```python
from build123d import *

# Parameters (mm, degrees)
F0_W          = 6
F0_H          = 3
F1_DEPTH      = 6
F2_DEPTH      = 2
F2_DEPTH_BACK = 3
F3_R          = 1.7
F4_DEPTH      = 4.8
F5_R          = 2
F6_R          = 1.7
F7_DEPTH      = 3


with BuildPart() as f1:
    # F0 (on Front) → F1 (new body, symmetric)
    with BuildSketch(Plane.XZ):
        with BuildLine():
            Line((10, 0), (22.5, 0))
            Line((22.5, 0), (18.9995524919, 20.0000000164))
            Line((18.9995524919, 20.0000000164), (18.9995524919, 25.5000000164))
            Line((18.9995524919, 25.5000000164), (8.0836130781, 25.5000000164))
            ThreePointArc((8.0836130781, 25.5000000164), (5.5476302699, 20.0983556377), (0, 17.8999996185))
            Line((0, 17.8999996185), (0, 15.5))
            Line((0, 15.5), (10, 15.5))
            Line((10, 15.5), (10, 0))
        make_face()
        with Locations((12.9995524922, 19.0000000164)):
            Rectangle(F0_W, F0_H, mode=Mode.SUBTRACT)
    extrude(amount=F1_DEPTH, both=True)

    # F0 (on Front) → F2 (join, two sides)
    with BuildSketch(Plane.XZ) as f2_sk:
        with BuildLine():
            ThreePointArc((0, 17.8999996185), (5.5476302699, 20.0983556377), (8.0836130781, 25.5000000164))
            Line((8.0836130781, 25.5000000164), (6.0785524919, 25.5000000164))
            ThreePointArc((6.0785524919, 25.5000000164), (4.1324570431, 21.5134004627), (0, 19.8999996185))
            Line((0, 19.8999996185), (0, 17.8999996185))
        make_face()
    extrude(amount=F2_DEPTH)
    extrude(f2_sk.sketch, amount=-F2_DEPTH_BACK)

    # F3 (on face) → F4 (cut)
    with BuildSketch(Plane.XY.offset(25.5000000164)):
        with Locations((12.9995524919, 0)):
            Circle(F3_R)
    extrude(amount=-F4_DEPTH, mode=Mode.SUBTRACT)

    # F5
    f5_edges = [f1.edges().sort_by_distance(p)[0] for p in [
        (20.749776, 6, 10),
        (18.999552, 6, 22.75),
        (20.749776, -6, 10),
        (18.999552, -6, 22.75),
    ]]
    fillet(f5_edges, radius=F5_R)

    # F6 (on face) → F7 (cut)
    with BuildSketch(Plane.XY.offset(17.5000000164)):
        with Locations((12.9995524922, 0)):
            Circle(F6_R)
    extrude(amount=-F7_DEPTH, mode=Mode.SUBTRACT)

    # F8: F1 across plane


with BuildPart() as f1_1:
    add(f1.part)
    add(f1.part.mirror(Plane.YZ))


solid = f1_1.part
```
Here's how the part is built. I have some questions about the finished solid (model axes, mm). A direction names the side the tool comes from. Coordinates: 2 decimals unless noted, no trailing zeros. Order: outer loops, then holes, each group sorted by start corner. A loop starts at its lowest first (then second) coordinate and runs counter-clockwise, first axis right, second up. Notation, with made-up numbers: M 17.5,78.25 L 39.5,78.25 A18 ccw 39.5,86.25 Z; hole C 39,-16 d11. An arc over 180 degrees is marked long. Answer as a JSON object with one key per item and string values. Group by question number.
(1) Suppose I cut it at C-C, the plane x = -5. Please give me the cut outline in (y, z), then the cut area to 3 significant figures.
(2) For pin 1 (1.7 mm diameter, centred on x = -13, y = -0.5, fed in from +Z); pin 2 (0.9 mm diameter, centred on y = -0.5, z = 19.5, fed in from -X); pin 3 (1 mm diameter, centred on x = -0.5, y = 0, fed in from +Z); pin 4 (3.5 mm diameter, centred on x = 12.5, y = 0.5, fed in from +Z), each with a flat end and sliding along its axis, tell me the tip position at first contact or that it passes through.
(3) Suppose I cut it at D-D, the plane y = 4.5. Please give me the cut outline in (x, z), then the cut area to 3 significant figures.
(4) Suppose I cut it at A-A, the plane y = -2.75. Please give me the cut outline in (x, z), then the cut area to 3 significant figures.
(5) Suppose I cut it at B-B, the plane z = 22.75. Please give me the cut outline in (x, y), then the cut area to 3 significant figures.
(6) Which directions (+Z, -Z, +X, -X, +Y, -Y) give clear straight access to the entire face, cutting with the end or side of a thin tool? Please do faces 1 (the face through (-13, 0, 14.5)), 2 (the face through (0, -2, 19)), 3 (the face through (10, 0, 8)), 4 (the face through (-16, 0, 19)), 5 (the face through (-19, 0, 23)).
(7) If we mould it in two halves opening along Y, with no side actions, what happens to faces 6 (the face through (20.12, 5.43, 10.12)), 7 (the face through (16, 0, 0)), 8 (the face through (13, 0, 20.7))? For each: released by +Y, released by -Y, zero draft, split by the parting line, or undercut.
(8) I need wall thicknesses on probe 1 along Z at (x, y) = (13, 5); probe 2 along X at (y, z) = (1.5, 15); probe 3 along X at (y, z) = (0.25, 22). Which ranges of each line are inside material? Lowest first, please.
Values found:
{
 "1": {"outline": "M -6,15.5 L 6,15.5 L 6,19.63 L 3,19.63 L 3,22.51 L -2,22.51 L -2,19.63 L -6,19.63 Z", "area": "63.9 mm^2"},
 "2": {"pin 1": "stops at z = 20.7", "pin 2": "stops at x = -19.17", "pin 3": "stops at z = 19.98", "pin 4": "stops at z = 25.5"},
 "3": {"outline": "M -22.44,0 L -10,0 L -10,15.5 L 10,15.5 L 10,0 L 22.44,0 L 18.94,19.99 L 18.94,25.5 L 8.08,25.5 A8.1 cw -8.08,25.5 L -18.94,25.5 L -18.94,19.99 Z; hole M -16,17.5 L -10,17.5 L -10,20.5 L -16,20.5 Z; hole M 10,17.5 L 16,17.5 L 16,20.5 L 10,20.5 Z", "area": "595 mm^2"},
 "4": {"outline": "M -22.5,0 L -10,0 L -10,15.5 L 10,15.5 L 10,0 L 22.5,0 L 19,20 L 19,25.5 L 8.08,25.5 A8.1 cw -8.08,25.5 L -19,25.5 L -19,20 Z; hole M -16,17.5 L -10,17.5 L -10,20.5 L -16,20.5 Z; hole M 10,17.5 L 16,17.5 L 16,20.5 L 10,20.5 Z", "area": "598 mm^2"},
 "5": {"outline": "M -19,-4 A2 ccw -17,-6 L -7.42,-6 L -7.42,-2 L -5.16,-2 L -5.16,3 L -7.42,3 L -7.42,6 L -17,6 A2 ccw -19,4 Z; M 5.16,-2 L 7.42,-2 L 7.42,-6 L 17,-6 A2 ccw 19,-4 L 19,4 A2 ccw 17,6 L 7.42,6 L 7.42,3 L 5.16,3 Z; hole C -13,0 d3.4; hole C 13,0 d3.4", "area": "279 mm^2"},
 "6": {"face 1": "none", "face 2": "+Z, -Y", "face 3": "-Z, +Y, -Y", "face 4": "+Y, -Y", "face 5": "+Z, -X, +Y, -Y"},
 "7": {"face 6": "released by +Y", "face 7": "zero draft", "face 8": "undercut"},
 "8": {"probe 1": "z = 0 to 17.5, 20.5 to 25.5", "probe 2": "x = -19.87 to -13.8, -12.2 to -10, 10 to 12.2, 13.8 to 19.87", "probe 3": "x = -19 to -14.68, -11.32 to -4.6, 4.6 to 11.32, 14.68 to 19"}
}
